The listing builds one solid part. Answer for the finished solid, in the listing's coordinates (mm). A direction names the side the tool comes from. Round coordinates to 2 decimals unless told otherwise and drop trailing zeros. Write each loop counter-clockwise with the first axis right and the second up, starting at its lowest first coordinate (ties: lowest second). Pieces come first, ordered by that corner, then holes.
from build123d import *

# Parameters (mm, degrees)
SKETCH2_R          = 0.8
CUT_EXTRUDE1_DEPTH = 4.8
CUT_EXTRUDE2_DEPTH = 4.8
CIRPATTERN1_COUNT  = 48
CUT_EXTRUDE3_DEPTH = 2.43
CIRPATTERN2_COUNT  = 11


with BuildPart() as part:
    # Sketch1 → Revolve1 (revolve)
    with BuildSketch(Plane.XY):
        Polygon((-6.2, 3.8), (-6.2, 2.43), (-2.65, 2.43), (-2.65, 0), (0, 0), (0, 3.8), align=None)
    revolve(axis=Axis((0, 3.8, 0), (0, -1, 0)))

    # Sketch2 → Cut-Extrude1 (cut, through all)
    with BuildSketch(Plane(origin=(0, 3.8, 0), x_dir=(1, 0, 0), z_dir=(0, 1, 0))):
        Circle(SKETCH2_R)
    extrude(amount=-CUT_EXTRUDE1_DEPTH, mode=Mode.SUBTRACT)

    # Sketch3 → Cut-Extrude2 (cut, through all)
    with BuildSketch(Plane(origin=(0, 3.8, 0), x_dir=(1, 0, 0), z_dir=(0, 1, 0))):
        with BuildLine():
            Line((0, 6.2), (0.364241202, 5.557246845))
            Line((0.364241202, 5.557246845), (0.809262392, 6.146958141))
            ThreePointArc((0.809262392, 6.146958141), (0.405499401, 6.186725324), (0, 6.2))
        make_face()
    cut_extrude2 = extrude(amount=-CUT_EXTRUDE2_DEPTH, mode=Mode.SUBTRACT)

    # CirPattern1: Cut-Extrude2 ×48 about axis
    cirpattern1_axis = Axis((0, 0, 0), (0, 1, 0))
    for i in range(1, CIRPATTERN1_COUNT):
        add(cut_extrude2.rotate(cirpattern1_axis, i * 360 / CIRPATTERN1_COUNT), mode=Mode.SUBTRACT)

    # Sketch4 → Cut-Extrude3 (cut)
    with BuildSketch(Plane.XZ):
        with BuildLine():
            Line((0, 2.65), (0.609443257, 2.075573123))
            Line((0.609443257, 2.075573123), (1.432698166, 2.229321862))
            ThreePointArc((1.432698166, 2.229321862), (0.746591276, 2.54265638), (0, 2.65))
        make_face()
    cut_extrude3 = extrude(amount=-CUT_EXTRUDE3_DEPTH, mode=Mode.SUBTRACT)

    # CirPattern2: Cut-Extrude3 ×11 about axis
    cirpattern2_axis = Axis((0, 0, 0), (0, 1, 0))
    for i in range(1, CIRPATTERN2_COUNT):
        add(cut_extrude3.rotate(cirpattern2_axis, i * 360 / CIRPATTERN2_COUNT), mode=Mode.SUBTRACT)


solid = part.part
1. A tool of negligible diameter and unlimited length cuts with its end or side. For faces 5 (the face through (-1.027, 1.198, 2.154)), 6 (the face through (0, 3.8, -1)), 7 (the face through (1.53, 1.2, 1.83)), 8 (the face through (1.592, 1.198, -1.777)), 9 (the face through (-3, 2.43, 0)), from which of +Z, -Z, +X, -X, +Y, -Y can it reach the whole face along a straight path? Write none if from no direction.
Geometry says:
face 5: +Z, -Y
face 6: +Z, -Z, +X, -X, +Y
face 7: +Z, +X, -Y
face 8: -Z, +X, -Y
face 9: -Y
2. Straight lines are drawn through the part: line 1 along Y through (x, z) = (-2.5, 2.5); line 2 along X through (y, z) = (1.3, 1); line 3 along X through (y, z) = (3.4, 4.75). For each, find the intervals that lie inside material, in ascending order.
Geometry says:
line 1: y = 2.43 to 3.8
line 2: x = -2.38 to 2.38
line 3: x = -3.75 to -3.38, -3.1 to 3.1, 3.38 to 3.75
3. Given pin 1 (2 mm diameter, centred on y = 3, z = 3, fed in from -X); pin 2 (1 mm diameter, centred on x = 4.5, y = 2.5, fed in from +Z); pin 3 (2 mm diameter, centred on x = -1.5, y = 2, fed in from -Z); pin 4 (2 mm diameter, centred on x = 0, z = 0, fed in from +Y), each flat-ended and moving along its own axis, determine where each tip first touches the part or whether it passes through.
Geometry says:
pin 1: stops at x = -5.73
pin 2: stops at z = 4.38
pin 3: stops at z = -6.15
pin 4: stops at y = 3.8
4. Section A-A on y = 1.6 is taken. Determine the outline of the cut face in (x, z), plus the area to 3 significant figures.
Geometry says:
outline: (-2.62, -0.38) - (-1.97, -0.9) - (-2, -1.74) - (-1.17, -1.82) - (-0.75, -2.54) - (0, -2.16) - (0.75, -2.54) - (1.17, -1.82) - (2, -1.74) - (1.97, -0.9) - (2.62, -0.38) - (2.14, 0.31) - (2.41, 1.1) - (1.63, 1.42) - (1.43, 2.23) - (0.61, 2.08) - (0, 2.65) - (-0.61, 2.08) - (-1.43, 2.23) - (-1.63, 1.42) - (-2.41, 1.1) - (-2.14, 0.31) - close; hole circle Ø1.6 at (0, 0)
area: 15.8 mm2
5. For a pull along Z with two mould halves and no side action, classify faces 1 (the face through (-1.58, 1.2, -1.78)), 2 (the face through (1.985, 1.198, -1.311)), 3 (the face through (-1.535, 1.198, 1.817)), 4 (the face through (-1.985, 1.198, -1.323)) as released by +Z, released by -Z, zero draft, split by the parting line, or undercut.
Geometry says:
face 1: released by -Z
face 2: undercut
face 3: released by +Z
face 4: undercut
